Can you work these out from the model? Positions are in its coordinate system, mm. Face numbers are marked on the shaded views. Round coordinates to 2 decimals unless told otherwise and drop trailing zeros. Write each loop counter-clockwise with the first axis right and the second up, starting at its lowest first coordinate (ties: lowest second). Pieces come first, ordered by that corner, then holes. Notation, with made-up numbers: M 29.25,20 L 43.25,20 A35 ccw 43.25,53 Z; hole C -11,-32 d9. An arc over 180 degrees is marked long. Answer in a Markdown table with one row per item. Add a question column.
(1) Suppose I cut it at B-B, the plane z = 8.5. Write out the boundary of the cut face in (x, y).
(2) Suppose I cut it at A-A, the plane x = 18.5. Write out the boundary of the cut face in (y, z), then the cut area to 3 significant figures.
(3) Suppose I cut it at D-D, the plane x = 39. Write out the boundary of the cut face in (y, z).
(4) Suppose I cut it at C-C, the plane y = -15.75. Write out the boundary of the cut face in (x, z), then the cut area to 3 significant figures.
(5) If I drill on probe 1 along Y at (x, z) = (12.7, 5.5); probe 2 along Z at (x, y) = (42, -12); probe 3 along X at (y, z) = (-14, 13.75), over which ranges is the centre line in solid material (lowest first)?
(6) I'm going to push flat-ended pins straight in: pin 1 (6 mm diameter, centred on x = 7.5, z = 13, fed in from +Y); pin 2 (3 mm diameter, centred on x = 35, y = -3, fed in from +Z); pin 3 (1.5 mm diameter, centred on y = -5, z = 10.5, fed in from +X); pin 4 (11.5 mm diameter, centred on x = 12.7, y = -12.7, fed in from -Z). Where does each tip first touch, or does it pass through?
(7) If we mould it in two halves opening along X, with no side actions, what happens to the marked faces 1, 2 and 3? For each: released by +X, released by -X, zero draft, split by the parting line, or undercut.
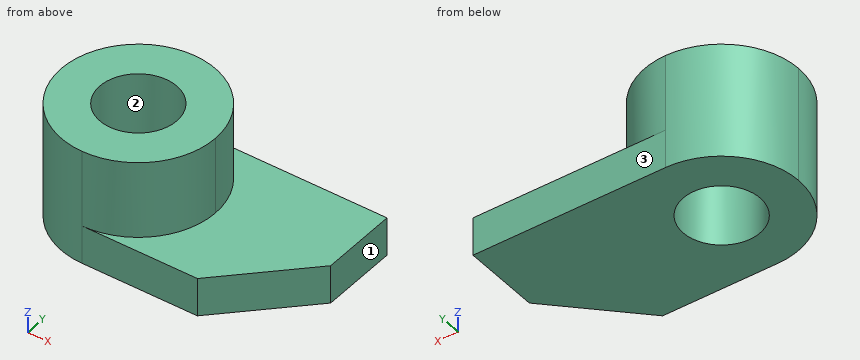
from build123d import *

# Parameters (mm, degrees)
F1_DEPTH = 6.35
F0_R     = 6.35
F2_DEPTH = 19.05
F4_DEPTH = 19.051


with BuildPart() as f1:
    # F0 (on Top) → F1 (new body)
    with BuildSketch(Plane.XY):
        with BuildLine():
            Line((44.45, 0), (12.7, 0))
            ThreePointArc((12.7, 0), (21.680256, -3.719744), (25.4, -12.7))
            ThreePointArc((25.4, -12.7), (21.680256, -21.680256), (12.7, -25.4))
            Line((12.7, -25.4), (44.45, -25.4))
            Line((44.45, -25.4), (44.45, 0))
        make_face()
    extrude(amount=F1_DEPTH)

    # F0 (on Top) → F2 (join)
    with BuildSketch(Plane.XY):
        with BuildLine():
            ThreePointArc((25.4, -12.7), (21.680256, -3.719744), (12.7, 0))
            ThreePointArc((12.7, 0), (3.719744, -3.719744), (0, -12.7))
            ThreePointArc((0, -12.7), (3.719744, -21.680256), (12.7, -25.4))
            ThreePointArc((12.7, -25.4), (21.680256, -21.680256), (25.4, -12.7))
        make_face()
        with Locations((12.7, -12.7)):
            Circle(F0_R, mode=Mode.SUBTRACT)
    extrude(amount=F2_DEPTH)

    # F3 (on Top) → F4 (cut, through all)
    with BuildSketch(Plane.XY):
        Polygon((44.45, -12.7), (31.75, -25.4), (44.45, -25.4), align=None)
    extrude(amount=F4_DEPTH, mode=Mode.SUBTRACT)


solid = f1.part
Calculated:
| question | item | result |
|---|---|---|
| 1 | outline | C 12.7,-12.7 d25.4; hole C 12.7,-12.7 d12.7 |
| 2 | outline | M -25.4,0 L -15.29,0 L -15.29,19.05 L -24,19.05 L -24,6.35 L -25.4,6.35 Z; M -10.11,0 L 0,0 L 0,6.35 L -1.4,6.35 L -1.4,19.05 L -10.11,19.05 Z |
| 2 | area | 350 mm² |
| 3 | outline | M -18.15,0 L 0,0 L 0,6.35 L -18.15,6.35 Z |
| 4 | outline | M 0.37,0 L 7.13,0 L 7.13,19.05 L 0.37,19.05 Z; M 18.27,0 L 41.4,0 L 41.4,6.35 L 25.03,6.35 L 25.03,19.05 L 18.27,19.05 Z |
| 4 | area | 361 mm² |
| 5 | probe 1 | -25.4 to -19.05, -6.35 to 0 |
| 5 | probe 2 | 0 to 6.35 |
| 5 | probe 3 | 0.07 to 6.48, 18.92 to 25.33 |
| 6 | pin 1 | y = -0.19 |
| 6 | pin 2 | z = 6.35 |
| 6 | pin 3 | x = 23.33 |
| 6 | pin 4 | through |
| 7 | face 1 | released by +X |
| 7 | face 2 | undercut |
| 7 | face 3 | zero draft |
